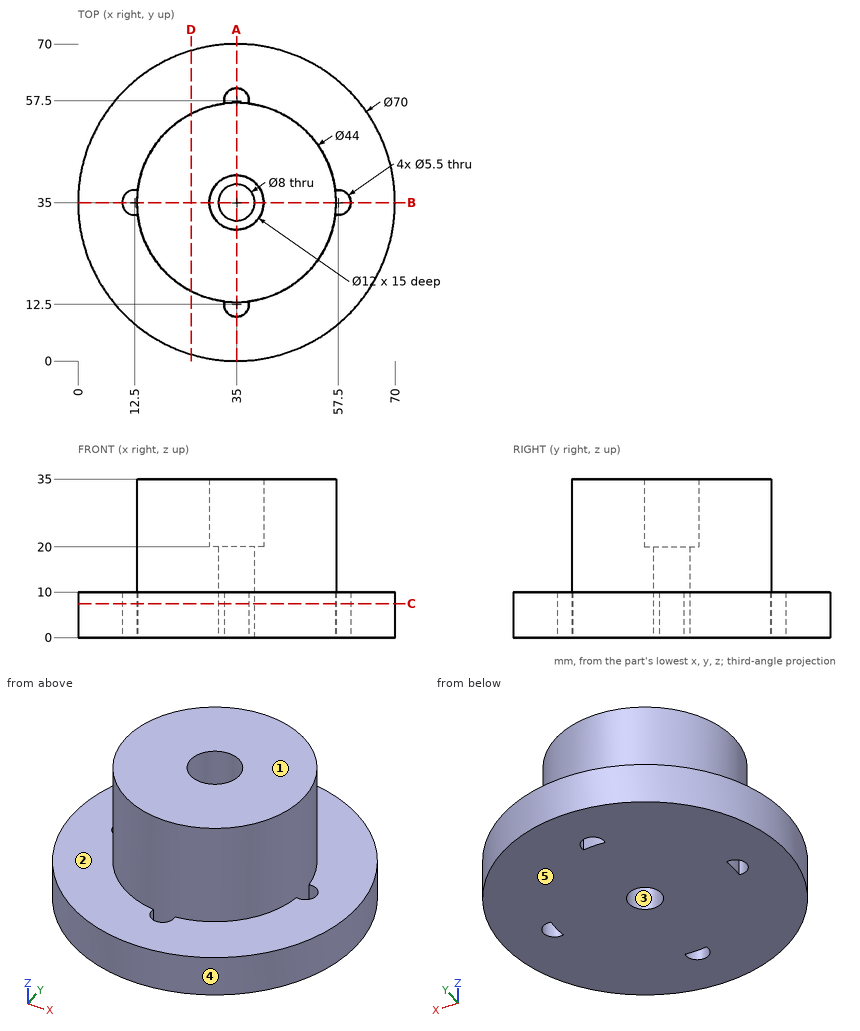
Here's the drawing with two shaded views (mm, measured from the low corner). I have some questions. A direction names the side the tool comes from. Coordinates: 2 decimals unless noted, no trailing zeros. Loops run counter-clockwise (first coordinate to the right, second up) from the corner with the lowest first, then second, coordinate; pieces in that order, holes last.
Item 1: Please list where these lines run through material, in increasing order: L1, parallel to Y at x = 35, z = 5.5; L2, parallel to X at y = 35, z = 24.75; L3, parallel to Z at x = 23, y = 15.
Answers below:
L1: y = 0 to 9.75, 13 to 31, 39 to 57, 60.25 to 70
L2: x = 13 to 29, 41 to 57
L3: z = 0 to 10
Item 2: Suppose I cut it at C-C (z = 7.5). Please give me the cut outline in (x, y), then the cut area to 3 significant figures.
Answers below:
outline: circle Ø70 at (35, 35); hole (13.16, 32.33) arc R22 cw to (13.16, 37.67) arc R2.75 ccw (long way) to start; hole circle Ø8 at (35, 35); hole (32.33, 13.16) arc R2.75 ccw (long way) to (37.67, 13.16) arc R22 cw to start; hole (32.33, 56.84) arc R22 cw to (37.67, 56.84) arc R2.75 ccw (long way) to start; hole (56.84, 32.33) arc R2.75 ccw (long way) to (56.84, 37.67) arc R22 cw to start
area: 3,740 mm2
Item 3: Suppose I cut it at D-D (x = 25). Please give me the cut outline in (y, z).
Answers below:
outline: (1.46, 0) - (68.54, 0) - (68.54, 10) - (54.6, 10) - (54.6, 35) - (15.4, 35) - (15.4, 10) - (1.46, 10) - close
Item 4: Which directions (+Z, -Z, +X, -X, +Y, -Y) give clear straight access to the entire face, cutting with the end or side of a thin tool? Please do the marked faces 1 and 2.
Answers below:
face 1: +Z, +X, -X, +Y, -Y
face 2: +Z
Item 5: Suppose I cut it at A-A (x = 35). Please give me the cut outline in (y, z), then the cut area to 4 significant figures.
Answers below:
outline: (0, 0) - (9.75, 0) - (9.75, 10) - (0, 10) - close; (13, 0) - (31, 0) - (31, 20) - (29, 20) - (29, 35) - (13, 35) - close; (39, 0) - (57, 0) - (57, 35) - (41, 35) - (41, 20) - (39, 20) - close; (60.25, 0) - (70, 0) - (70, 10) - (60.25, 10) - close
area: 1,395 mm2
Item 6: If we mould it in two halves opening along X, with no side actions, what happens to the marked faces 3, 4 and 5? For each: released by +X, released by -X, zero draft, split by the parting line, or undercut.
Answers below:
face 3: undercut
face 4: split by the parting line
face 5: zero draft
Item 7: I'm going to push flat-ended pins straight in: pin 1 (7 mm diameter, centred on x = 35, y = 35, fed in from +Z); pin 2 (3 mm diameter, centred on x = 32, y = 10, fed in from +Z); pin 3 (3 mm diameter, centred on y = 36.5, z = 21, fed in from +X); pin 4 (6 mm diameter, centred on x = 56.5, z = 14, fed in from -Y). Where does each tip first touch, or does it pass through?
Answers below:
pin 1: passes through
pin 2: stops at z = 10
pin 3: stops at x = 57
pin 4: stops at y = 23.09
